Geometry: final body of the model. Coordinates: model frame, mm. Give positions to 0.01 mm unless a question says otherwise; leave off trailing zeros. Write each loop counter-clockwise with the first axis right and the second up, starting at its lowest first coordinate (ties: lowest second). Pieces come first, ordered by that corner, then holes. Notation, with made-up numbers: (89, 30) - (132, 30) arc R18 cw to (132, 43) - close; hole circle Ø10 at (9.5, 54.25). An arc over 180 degrees is marked (long way). Return JSON: item names as keys, results as strings.
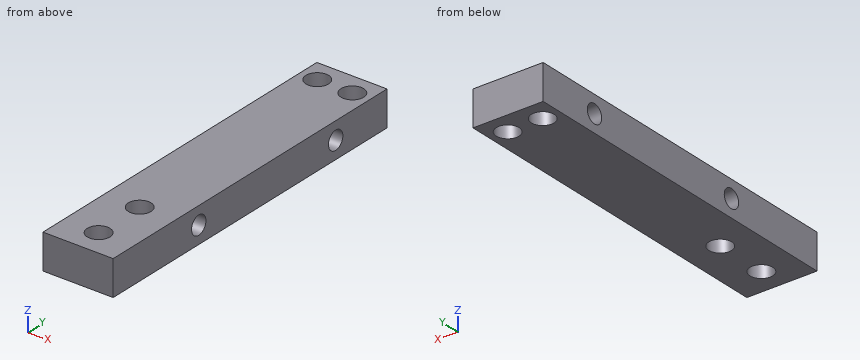
from build123d import *

# Parameters (mm, degrees)
F0_W          = 16
F0_H          = 8
F1_DEPTH      = 80
F2_R          = 2.6
F4_DEPTH      = 25
F4_DEPTH_BACK = 25
F5_D          = 4.2
F5_DEPTH      = 18.4
F5_TIP        = 1.2618073


with BuildPart() as f1:
    # F0 (on Front) → F1 (new body)
    with BuildSketch(Plane.XZ):
        Rectangle(F0_W, F0_H)
    extrude(amount=-F1_DEPTH)

    # F2 (on face) → F4 (cut, two sides)
    with BuildSketch(Plane.XY.offset(4)) as f4_sk:
        with Locations((0, 18)):
            Circle(F2_R)
        with Locations((0, 6)):
            Circle(F2_R)
        with Locations((4, 75)):
            Circle(F2_R)
        with Locations((-4, 75)):
            Circle(F2_R)
    extrude(amount=-F4_DEPTH, mode=Mode.SUBTRACT)
    extrude(f4_sk.sketch, amount=F4_DEPTH_BACK, mode=Mode.SUBTRACT)

    # F5
    with Locations(Plane(origin=(-8, 0, 0), x_dir=(0, -1, 0), z_dir=(-1, 0, 0))):
        with Locations((-65, 0), (-25, 0)):
            Hole(F5_D / 2, depth=F5_DEPTH)
            with Locations((0, 0, -(F5_DEPTH + F5_TIP / 2))):  # 118° drill point
                Cone(0, F5_D / 2, F5_TIP, mode=Mode.SUBTRACT)


solid = f1.part
Q1. Section query A-A, the plane y = 65. Return the cut outline in (x, z).
Answer key:
{"outline": "(-8, -4) - (8, -4) - (8, -2.1) - (-8, -2.1) - close; (-8, 2.1) - (8, 2.1) - (8, 4) - (-8, 4) - close"}
Q2. Section query C-C, the plane z = 3. Return the cut outline in (x, y).
Answer key:
{"outline": "(-8, 0) - (8, 0) - (8, 80) - (-8, 80) - close; hole circle Ø5.2 at (-4, 75); hole circle Ø5.2 at (0, 6); hole circle Ø5.2 at (0, 18); hole circle Ø5.2 at (4, 75)"}
Q3. Section query B-B, the plane x = 0. Return the cut outline in (y, z).
Answer key:
{"outline": "(0, -4) - (3.4, -4) - (3.4, 4) - (0, 4) - close; (8.6, -4) - (15.4, -4) - (15.4, 4) - (8.6, 4) - close; (20.6, -4) - (80, -4) - (80, 4) - (20.6, 4) - close; hole circle Ø4.2 at (25, 0); hole circle Ø4.2 at (65, 0)"}
Q4. Material intervals for probe 1 along Y at (x, z) = (0, -0.25); probe 2 along Y at (x, z) = (5, 1.75); probe 3 along Y at (x, z) = (-7, 0.5), sorted ascending. Write a range as [from, to].
Answer key:
{"probe 1": "y = [0, 3.4], [8.6, 15.4], [20.6, 22.91], [27.09, 62.91], [67.09, 80]", "probe 2": "y = [0, 23.84], [26.16, 63.84], [66.16, 72.6], [77.4, 80]", "probe 3": "y = [0, 22.96], [27.04, 62.96], [67.04, 80]"}
Q5. Section query D-D, the plane y = 75. Return the cut outline in (x, z).
Answer key:
{"outline": "(-8, -4) - (-6.6, -4) - (-6.6, 4) - (-8, 4) - close; (-1.4, -4) - (1.4, -4) - (1.4, 4) - (-1.4, 4) - close; (6.6, -4) - (8, -4) - (8, 4) - (6.6, 4) - close"}
Q6. Pin query (flat end, axial travel): P1, Ø6, axis at x = -4, y = 75, coming from the -Z side. Return the tip coordinate at first contact, or that it passes through.
Answer key:
{"P1": "stops at z = -4"}
